Study the drawing (mm; zero at the part's minimum x, y, z) and answer. A direction names the side the tool comes from. Round coordinates to 2 decimals unless told otherwise and drop trailing zeros. Order: outer loops, then holes, each group sorted by start corner. A loop starts at its lowest first (then second) coordinate and runs counter-clockwise, first axis right, second up. Notation, with made-up numbers: (9, -5.5) - (50, -5.5) arc R14 cw to (50, 4.5) - close; hole circle Ø2 at (86, 24.25). An arc over 180 degrees is marked (long way). Put each result on its own line as item: value.
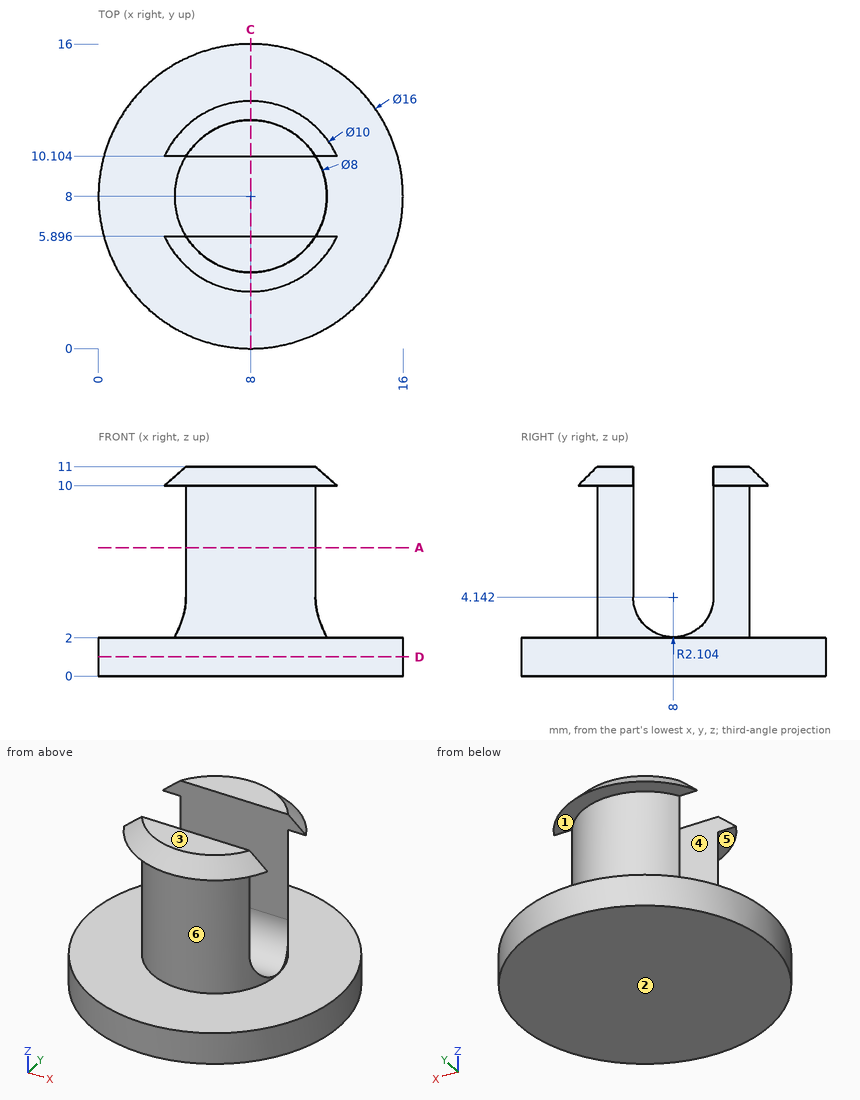
1) A cutting plane is placed at D-D on z = 1. Write down the section's boundary in (x, y).
Findings below:
outline: circle Ø16 at (8, 8)
2) Given pin 1 Ø3.5 at (x, z) = (9.5, 8) entering from -Y; pin 2 Ø2 at (x, z) = (7, 5) entering from +Y; pin 3 Ø4 at (x, y) = (4.5, 14) entering from +Z (1 decimal), each flat-ended and moving along its own axis, determine where each tip first touches the part or whether it passes through.
Findings below:
pin 1: stops at y = 4
pin 2: stops at y = 12
pin 3: stops at z = 10.1
3) Straight lines are drawn through the part: L1, parallel to Z at x = 4.5, y = 3.75; L2, parallel to Y at x = 7.5, z = 4; L3, parallel to Z at x = 10.5, y = 4 (1 decimal). For each, find the intervals that lie inside material, in ascending order. Write a range as from..to.
Findings below:
L1: z = 0..2
L2: y = 4.03..5.9, 10.1..11.97
L3: z = 0..2, 10..10.3
4) A cutting plane is placed at A-A on z = 6.75. Write down the section's boundary in (x, y).
Findings below:
outline: (4.6, 5.9) arc R4 ccw to (11.4, 5.9) - close; (4.6, 10.1) - (11.4, 10.1) arc R4 ccw to start
5) A cutting plane is placed at C-C on x = 8. Write down the section's boundary in (y, z).
Findings below:
outline: (0, 0) - (16, 0) - (16, 2) - (12, 2) - (12, 10) - (13, 10) - (12, 11) - (10.1, 11) - (10.1, 4.14) arc R2.1 cw to (5.9, 4.14) - (5.9, 11) - (4, 11) - (3, 10) - (4, 10) - (4, 2) - (0, 2) - close
6) For the marked faces 4, 5 and 6, determine the directions among +Z, -Z, +X, -X, +Y, -Y from which every point of the face is accessible in a straight line to the end or side of a thin tool.
Findings below:
face 4: +Z, +X, -X
face 5: -Y
face 6: none
7) For a pull along Z with two mould halves and no side action, classify the marked faces 1, 2 and 3 as pulls with the +Z half, pulls with the -Z half, needs draft (parallel to the pull), parting line crosses it, or undercut.
Findings below:
face 1: undercut
face 2: pulls with the -Z half
face 3: pulls with the +Z half
